Job drawing, mm, ordinate dimensions from the low corner. One solid piece. A direction names the side the tool comes from. Coordinates: 2 decimals unless noted, no trailing zeros. Loops run counter-clockwise (first coordinate to the right, second up) from the corner with the lowest first, then second, coordinate; pieces in that order, holes last. Notation, with made-up numbers: M 79.25,11.5 L 101.25,11.5 A31 cw 101.25,44.5 Z; hole C -26.75,62.25 d10. An arc over 180 degrees is marked long. Write each question's results on one line, items separated by ' | '. Start each with the question number.
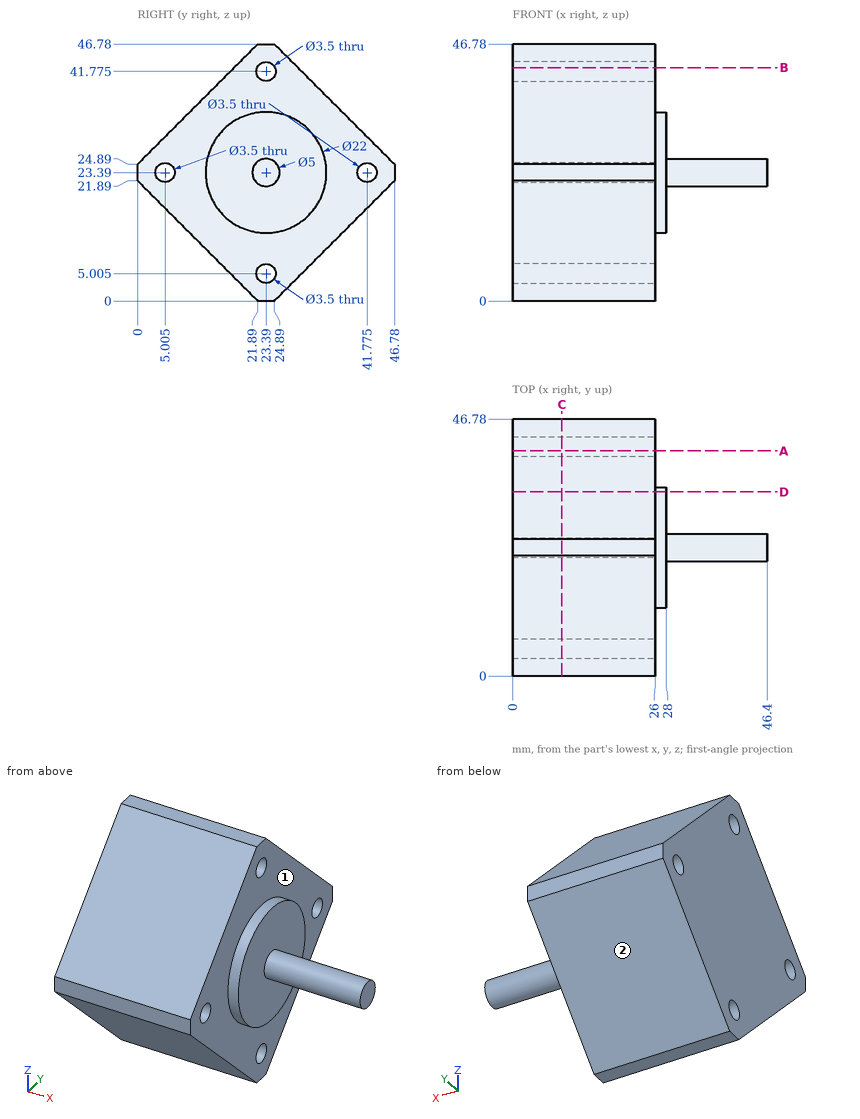
1. Band-saw the part on D-D, the plane y = 33.5. List the corners of the cut face in (x, z) (1 decimal).
2. Band-saw the part on C-C, the plane x = 9. Give the number of separate pieces and of enclosed holes in the cut face, plus the area to 3 significant figures.
3. Which spindle directions (+Z, -Z, +X, -X, +Y, -Y) get a long thin tool onto all of the face, cutting with end or side? Do the marked faces 1 and 2. Say none if no direction does.
4. Wall check: line 1 along X through (y, z) = (28.5, 30.5); line 2 along X through (y, z) = (20, 39); line 3 along Z through (x, y) = (17.5, 6). Give the ranges that are in metal, low to high.
5. Pin check, flat tips, straight feed: pin 1 (4 mm diameter, centred on x = 13.5, y = 37, fed in from +Z); pin 2 (4 mm diameter, centred on y = 13.5, z = 24, fed in from +X); pin 3 (5.5 mm diameter, centred on y = 41.77, z = 23.39, fed in from +X). Stop position of each tip, or through.
6. Band-saw the part on A-A, the plane y = 41. List the corners of the cut face in (x, z).
7. Band-saw the part on B-B, the plane z = 42.5. List the corners of the cut face in (x, y), plus the area to 3 significant figures.
Checked values:
1) outline: M 0,8.6 L 26,8.6 L 26,19.1 L 28,19.1 L 28,27.7 L 26,27.7 L 26,38.2 L 0,38.2 Z
2) separate pieces: 1 | enclosed holes: 4 | area: 1,190 mm²
3) face 1: +X | face 2: -Z, +X, -X, +Y
4) line 1: 0 to 28 | line 2: 0 to 26 | line 3: 15.89 to 21.95, 24.83 to 30.89
5) pin 1: z = 36.67 | pin 2: x = 28 | pin 3: x = 26
6) outline: M 0,16.11 L 26,16.11 L 26,21.82 L 0,21.82 Z; M 0,24.96 L 26,24.96 L 26,30.67 L 0,30.67 Z
7) outline: M 0,17.61 L 26,17.61 L 26,21.8 L 0,21.8 Z; M 0,24.98 L 26,24.98 L 26,29.17 L 0,29.17 Z | area: 218 mm²
